Input: part model. Units: mm. Frame: model coordinates. Face numbers are marked on the shaded views. A direction names the side the tool comes from. Give positions to 0.01 mm unless a question says otherwise; leave off trailing zeros. Write each loop counter-clockwise with the first axis right and the second up, starting at its lowest first coordinate (ties: lowest second). Pieces come first, ordered by that corner, then holes. Notation, with made-up numbers: (-6.5, 82.25) -> (2.5, 82.25) arc R33 ccw to (2.5, 118.25) -> close; hole circle Ø2 at (2, -35). An arc over 180 degrees is marked (long way). Answer as a JSON object with one key per item and string values. Group by question number.
from build123d import *

# Parameters (mm, degrees)
SKETCH_1_W          = 64.5
SKETCH_1_H          = 47.5
EXTRUDE_1_DEPTH     = 2.6
FILLET_1_R          = 12.5
SKETCH_2_R          = 1.5
SKETCH_2_R_2        = 1.75
SKETCH_2_W          = 2.7
SKETCH_2_H          = 5.4
SKETCH_2_W_2        = 15.5
SKETCH_2_H_2        = 10.5
CUT_EXTRUDE_1_DEPTH = 2.6
SKETCH_3_R          = 4.6
SKETCH_3_R_2        = 2.75
EXTRUDE_2_DEPTH     = 5
CUT_EXTRUDE_START   = -26
SKETCH_4_R          = 1.5
CUT_EXTRUDE_2_DEPTH = 26


with BuildPart() as part:
    # 草图1 → 凸台-拉伸1 (new body)
    with BuildSketch(Plane.XY):
        Rectangle(SKETCH_1_W, SKETCH_1_H)
    extrude(amount=EXTRUDE_1_DEPTH)

    # 圆角1
    fillet_1_edges = [part.edges().sort_by_distance(p)[0] for p in [
        (-32.25, 23.75, 1.3),
        (32.25, 23.75, 1.3),
    ]]
    fillet(fillet_1_edges, radius=FILLET_1_R)

    # 草图2 → 切除-拉伸1 (cut)
    with BuildSketch(Plane.XY.offset(2.6)):
        with Locations((-19.25, -10.75)):
            Circle(SKETCH_2_R)
        with Locations((-28.75, 8.75)):
            Circle(SKETCH_2_R)
        with Locations((27.75, -8.25)):
            Circle(SKETCH_2_R_2)
        with Locations((23.75, -1.25)):
            Circle(SKETCH_2_R)
        with Locations((9.75, -1.25)):
            Circle(SKETCH_2_R)
        with Locations((-3.75, 13.25)):
            Circle(SKETCH_2_R_2)
        with Locations((-10.9, -17.05)):
            Rectangle(SKETCH_2_W, SKETCH_2_H)
        with Locations((16.5, -10.7)):
            Rectangle(SKETCH_2_W_2, SKETCH_2_H_2)
    extrude(amount=-CUT_EXTRUDE_1_DEPTH, mode=Mode.SUBTRACT)

    # 草图3 → 凸台-拉伸2 (add)
    with BuildSketch(Plane.XY.offset(2.6)):
        with Locations((-19.75, 11.25)):
            Circle(SKETCH_3_R)
        with Locations(Location((19.75, 11.25, 0), (0, 0, 180))):
            Circle(SKETCH_3_R)
        with Locations((9.75, -1.25)):
            Circle(SKETCH_3_R_2)
        with Locations((23.75, -1.25)):
            Circle(SKETCH_3_R_2)
    extrude(amount=EXTRUDE_2_DEPTH)

    # 草图4 → 切除-拉伸2 (cut)
    with BuildSketch(Plane(origin=(0, 0, 0), x_dir=(-1, 0, 0), z_dir=(0, 0, -1)).offset(CUT_EXTRUDE_START)):
        with Locations(Location((-23.75, -1.25, 0), (0, 0, 180))):
            Circle(SKETCH_4_R)
        with Locations(Location((-9.75, -1.25, 0), (0, 0, 180))):
            Circle(SKETCH_4_R)
    extrude(amount=CUT_EXTRUDE_2_DEPTH, mode=Mode.SUBTRACT)


solid = part.part
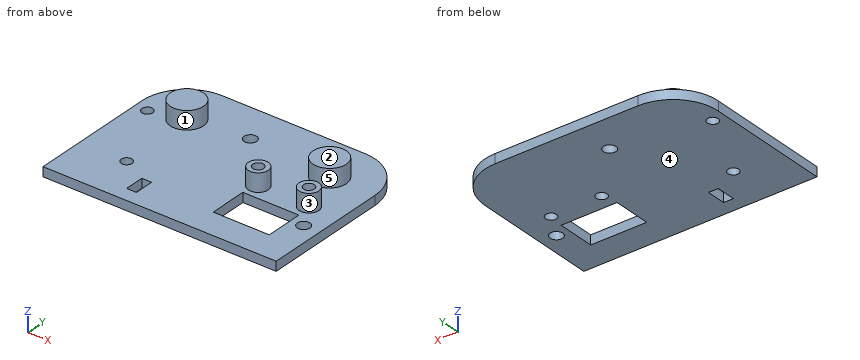
1. Section A-A (x = -3.75). Return the cut outline in (y, z).
2. Section C-C (x = 9.75). Return the cut outline in (y, z).
3. Section D-D (y = -1.25). Return the cut outline in (x, z).
4. Line query: line 1 (X direction, y = -6, z = 1.25); line 2 (X direction, y = -0.5, z = 4.25); line 3 (Z direction, x = 8, y = -5). Output: solid intervals per line, ascending.
5. Mould query, pull axis X, two halves, no side actions, for the marked faces 1, 2 and 3. Classes: pulls with the +X half, pulls with the -X half, needs draft (parallel to the pull), parting line crosses it, or undercut.
6. Reachability of the marked faces 4 and 5 from +Z, -Z, +X, -X, +Y, -Y: full face, straight path, thin tool, end or side. Return the list, or none.
7. Section B-B (z = 4.25). Return the cut outline in (x, y).
Working result:
{
 "1": {"outline": "(-23.75, 0) -> (11.5, 0) -> (11.5, 2.6) -> (-23.75, 2.6) -> close; (15, 0) -> (23.75, 0) -> (23.75, 2.6) -> (15, 2.6) -> close"},
 "2": {"outline": "(-23.75, 0) -> (-15.95, 0) -> (-15.95, 2.6) -> (-23.75, 2.6) -> close; (-5.45, 0) -> (-2.75, 0) -> (-2.75, 7.6) -> (-4, 7.6) -> (-4, 2.6) -> (-5.45, 2.6) -> close; (0.25, 0) -> (23.75, 0) -> (23.75, 2.6) -> (1.5, 2.6) -> (1.5, 7.6) -> (0.25, 7.6) -> close"},
 "3": {"outline": "(-32.25, 0) -> (8.25, 0) -> (8.25, 7.6) -> (7, 7.6) -> (7, 2.6) -> (-32.25, 2.6) -> close; (11.25, 0) -> (22.25, 0) -> (22.25, 7.6) -> (21, 7.6) -> (21, 2.6) -> (12.5, 2.6) -> (12.5, 7.6) -> (11.25, 7.6) -> close; (25.25, 0) -> (32.25, 0) -> (32.25, 2.6) -> (26.5, 2.6) -> (26.5, 7.6) -> (25.25, 7.6) -> close"},
 "4": {"line 1": "x = -32.25 to 8.75, 24.25 to 32.25", "line 2": "x = 7.1 to 8.45, 11.05 to 12.4, 21.1 to 22.45, 25.05 to 26.4", "line 3": "z = 0 to 2.6"},
 "5": {"face 1": "undercut", "face 2": "needs draft", "face 3": "undercut"},
 "6": {"face 4": "-Z, +X, -X, +Y, -Y", "face 5": "+Z"},
 "7": {"outline": "circle Ø9.2 at (-19.75, 11.25); circle Ø5.5 at (9.75, -1.25); circle Ø9.2 at (19.75, 11.25); circle Ø5.5 at (23.75, -1.25); hole circle Ø3 at (9.75, -1.25); hole circle Ø3 at (23.75, -1.25)"}
}
